Part model, mm, in its own coordinate system. A direction names the side the tool comes from. Give positions to 0.01 mm unless a question says otherwise; leave off trailing zeros. Loops run counter-clockwise (first coordinate to the right, second up) from the corner with the lowest first, then second, coordinate; pieces in that order, holes last. Notation, with made-up numbers: M 35,-7.75 L 46,-7.75 A7 cw 46,5.25 Z; hole C 51.25,65 d4. An arc over 180 degrees is marked long. Put each result on its own line as item: value. Start each with the question number.
Autodesk Inventor part; units mm, degrees
ref_plane "YZ Plane" through (0, 0, 0) normal (1, 0, 0) x (0, 1, 0)
ref_plane "XZ Plane" through (0, 0, 0) normal (0, 1, 0) x (-1, 0, 0)
ref_plane "XY Plane" through (0, 0, 0) normal (0, 0, 1) x (1, 0, 0)
sketch "Szkic1" plane through (0, 0, 0) normal (0, 1, 0) x (-1, 0, 0)
  line L0 (-8, 20) -> (13, 20)
  line L1 (13, 20) -> (13, -20)
  line L2 (13, -20) -> (-8, -20)
  line L3 (-13, 20) -> (13, -20) construction
  line L4 (13, 20) -> (-13, -20) construction
  line L5 (13, 0) -> (0, 0)
  circle A0 centre (0, 0) radius 5
  line L6 (13, 20) -> (-8, 20)
  arc A1 (-8, 10.247) -> (-8, -10.247) centre (0, 0) ccw
  line L7 (-8, 20) -> (-8, 10.247)
  line L8 (-8, -10.247) -> (-8, -20)
  dimension "d0" = 26
  dimension "d1" = 40
  dimension "d2" = 10
  dimension "d3" = 21
extrude "Wyciągnięcie proste1" add sketch "Szkic1" along normal blind 68
sketch "Szkic2" plane through (0, 68, 0) normal (0, 1, 0) x (1, 0, 0)
  circle A0 centre (0, 0) radius 5
  circle A1 centre (0, 0) radius 6
  circle A2 centre (0, 0) radius 10.5
  circle A3 centre (0, 0) radius 9.5
  dimension "d6" = 12
  dimension "d7" = 21
  dimension "d8" = 19
extrude "Wyciągnięcie proste2" cut sketch "Szkic2" against normal blind 1
sketch "Szkic3" plane through (0, 68, 0) normal (0, 1, 0) x (1, 0, 0)
  circle A0 centre (0, 0) radius 6
  circle A1 centre (0, 0) radius 9.5
extrude "Wyciągnięcie proste3" cut sketch "Szkic3" against normal blind 2
sketch "Szkic4" plane through (0, 0, 0) normal (0, -1, 0) x (1, 0, 0)
  circle A0 centre (0, 0) radius 5
  circle A1 centre (0, 0) radius 6
  circle A2 centre (0, 0) radius 10.5
  circle A3 centre (0, 0) radius 9.5
  dimension "d13" = 12
  dimension "d14" = 21
  dimension "d15" = 19
extrude "Wyciągnięcie proste4" cut sketch "Szkic4" against normal blind 1
sketch "Szkic5" plane through (0, 0, 0) normal (0, -1, 0) x (1, 0, 0)
  circle A0 centre (0, 0) radius 6
  circle A1 centre (0, 0) radius 9.5
extrude "Wyciągnięcie proste5" cut sketch "Szkic5" against normal blind 2
sketch "Szkic6" plane through (-13, 0, -20) normal (-1, 0, 0) x (0, 0, 1)
  line L0 (0, 0) -> (40, 0)
  line L1 (40, 0) -> (40, 68)
  line L2 (0, 68) -> (40, 68)
  line L3 (0, 0) -> (0, 68)
  line L4 (0, 68) -> (20, 68)
  line L5 (20, 68) -> (6, 68)
  line L6 (20, 68) -> (34, 68)
  line L7 (34, 68) -> (34, 0)
  line L8 (0, 0) -> (40, 0)
  line L9 (6, 68) -> (6, 0)
  line L10 (34, 68) -> (34, 34)
  line L11 (34, 34) -> (6, 34)
  line L12 (34, 34) -> (34, 57)
  line L13 (34, 57) -> (6, 57)
  line L14 (6, 34) -> (6, 11)
  line L15 (6, 11) -> (34, 11)
  point P0 (20, 0)
  dimension "d20" = 20
  dimension "d21" = 14
  dimension "d22" = 14
  dimension "d23" = 34
  dimension "d24" = 23
  dimension "d25" = 23
hole "Otwór1" at (-13, 57, -14) at (-13, 57, 14) at (-13, 11, -14) at (-13, 11, 14) direction (1, 0, 0) diameter 5 depth 12 tip angle 118
thread "Gwint1"
thread "Gwint2"
thread "Gwint3"
thread "Gwint4"
properties part number "Łożysko liniowe w obudowie SMAG10UU-L"
1) Pin check, flat tips, straight feed: pin 1 Ø10.5 at (x, z) = (1, 0.5) entering from -Y; pin 2 Ø2 at (y, z) = (39, -10) entering from +X; pin 3 Ø8 at (x, z) = (-8.5, 4) entering from -Y; pin 4 Ø5.5 at (x, z) = (-0.5, -4.5) entering from +Y. Stop position of each tip, or through.
2) Wall check: L1, parallel to Y at x = -5, z = 14; L2, parallel to Z at x = -10.5, y = 57; L3, parallel to Z at x = -2.5, y = 57. Give the ranges that are in metal, low to high.
3) Mould opens along Y. For faces 1 (the flat face through (-4, 1, 4)), 2 (the flat face through (-2, 34, 20)), 3 (the cylindrical face through (-6.92, 55.31, -15.84)), 4 (the flat face through (-0.1, 66, 6.2)) say: +Y half, -Y half, draft (parallel to the pull), parting line (faces both ways), or undercut.
4) Band-saw the part on C-C on x = -8.75. Give the cut face in (y, z).
5) Which spindle directions (+Z, -Z, +X, -X, +Y, -Y) get a long thin tool onto all of the face, cutting with end or side? Do faces 5 (the cylindrical face through (4.38, 66.51, 8.43)), 6 (the flat face through (-5, 1, -9)), 7 (the cylindrical face through (-6.9, 56.9, 11.5)). Say none if no direction does.
6) Band-saw the part on B-B on y = 22. Give the cut face in (x, z), then the cut area to 3 significant figures.
Evaluation:
1. pin 1: y = 1
1. pin 2: x = 9.38
1. pin 3: y = 0
1. pin 4: y = 67
2. L1: 0 to 8.5, 13.5 to 54.5, 59.5 to 68
2. L2: -20 to -16.5, -11.5 to 11.5, 16.5 to 20
2. L3: -20 to -16.5, -11.5 to -4.33, 4.33 to 11.5, 16.5 to 20
3. face 1: -Y half
3. face 2: draft
3. face 3: undercut
3. face 4: +Y half
4. outline: M 0,-20 L 68,-20 L 68,-5.8 L 67,-5.8 L 67,-3.7 L 66,-3.7 L 66,3.7 L 67,3.7 L 67,5.8 L 68,5.8 L 68,20 L 0,20 L 0,5.8 L 1,5.8 L 1,3.7 L 2,3.7 L 2,-3.7 L 1,-3.7 L 1,-5.8 L 0,-5.8 Z; hole C 11,-14 d5; hole C 11,14 d5; hole C 57,-14 d5; hole C 57,14 d5
5. face 5: +Y
5. face 6: -Y
5. face 7: -X
6. outline: M -13,-20 L 8,-20 L 8,-10.25 A13 ccw 8,10.25 L 8,20 L -13,20 Z; hole C 0,0 d10
6. area: 833 mm2
